Read the model definition and answer for the solid it produces. Units are mm, in the model's axes. A direction names the side the tool comes from. Coordinates: 2 decimals unless noted, no trailing zeros. Loops run counter-clockwise (first coordinate to the right, second up) from the corner with the lowest first, then second, coordinate; pieces in that order, holes last. Notation, with made-up numbers: (-18, 34.5) - (31, 34.5) arc R22 ccw to (31, 65.5) - close; hole circle Ø2 at (-6.75, -15). An arc over 180 degrees is marked (long way). Use one line per item in the form item = value. Start each with the question number.
1) A cutting plane is placed at C-C (z = 2.75). Give the vertices of the cut face in (x, y), and give its area (3 significant figures).
2) The mould has two halves that part along Y. Classify faces 4 (the face through (1, -1, 6.1)), 5 (the face through (-5.158, -3.955, 2.613)), 6 (the face through (0, -1, 3)): released by +Y, released by -Y, zero draft, split by the parting line, or undercut.
3) A cutting plane is placed at A-A (y = 0). Give the vertices of the cut face in (x, z).
4) Consider line 1 (Y direction, x = 0, z = 4); line 2 (Z direction, x = 2, y = -4.5); line 3 (X direction, y = 4.75, z = 1.5). Determine where each line is inside the solid, lowest interval first.
5) A cutting plane is placed at D-D (x = -5). Give the vertices of the cut face in (y, z), and give its area (3 significant figures).
6) Which of the six approach directions +Z, -Z, +X, -X, +Y, -Y give full straight-line access (tool end or side, diameter ignored) to faces 1 (the face through (3, 3, 0)), 2 (the face through (3, 3, 5.3)), 3 (the face through (1, 1, -0.8))?
7) Each of these flat-tipped pins is pushed along its axis until it touches: P1, Ø3, axis at x = 4, y = -3, coming from the +Z side; P2, Ø1, axis at x = 4.5, y = 1, coming from the -Z side; P3, Ø2, axis at x = 4, y = -5, coming from the +Z side. Where does it stop, or does it pass through?
from build123d import *

# Parameters (mm, degrees)
F0_R       = 6.5
F1_DEPTH   = 5.3
F2_R       = 4
F3_DEPTH   = 0.8
F4_R       = 4
F5_DEPTH   = 0.8
F6_SIZE2   = 0.6
F6_SIZE    = 2
F6_2_SIZE2 = 0.6
F6_2_SIZE  = 2
F7_R       = 1
F8_DEPTH   = 6.9


with BuildPart() as f1:
    # F0 (on Top) → F1 (new body)
    with BuildSketch(Plane.XY):
        Circle(F0_R)
    extrude(amount=F1_DEPTH)

    # F2 (on face) → F3 (join)
    with BuildSketch(Plane.XY.offset(5.3)):
        Circle(F2_R)
    extrude(amount=F3_DEPTH)

    # F4 (on face) → F5 (join)
    with BuildSketch(Plane(origin=(0, 0, 0), x_dir=(1, 0, 0), z_dir=(0, 0, -1))):
        Circle(F4_R)
    extrude(amount=F5_DEPTH)

    # F6
    f6_edges = [f1.edges().sort_by_distance(p)[0] for p in [
        (-4, 0, -0.8),
    ]]
    f6_side = f1.faces().sort_by_distance((0, 0, -0.8))[0]
    chamfer(f6_edges, length=F6_SIZE, length2=F6_SIZE2, reference=f6_side)

    # F6#2
    f6_2_edges = [f1.edges().sort_by_distance(p)[0] for p in [
        (-4, 0, 6.1),
    ]]
    f6_2_side = f1.faces().sort_by_distance((0, 0, 6.1))[0]
    chamfer(f6_2_edges, length=F6_2_SIZE, length2=F6_2_SIZE2, reference=f6_2_side)

    # F7 (on face) → F8 (cut, through all)
    with BuildSketch(Plane.XY.offset(6.1)):
        Circle(F7_R)
    extrude(amount=-F8_DEPTH, mode=Mode.SUBTRACT)


solid = f1.part
Found:
q1.outline = circle Ø13 at (0, 0); hole circle Ø2 at (0, 0)
q1.area = 130 mm^2
q2.face_4 = zero draft
q2.face_5 = split by the parting line
q2.face_6 = undercut
q3.outline = (-6.5, 0) - (-4, 0) - (-4, -0.2) - (-2, -0.8) - (-1, -0.8) - (-1, 6.1) - (-2, 6.1) - (-4, 5.5) - (-4, 5.3) - (-6.5, 5.3) - close; (1, -0.8) - (2, -0.8) - (4, -0.2) - (4, 0) - (6.5, 0) - (6.5, 5.3) - (4, 5.3) - (4, 5.5) - (2, 6.1) - (1, 6.1) - close
q4.line_1 = -6.5 to -1, 1 to 6.5
q4.line_2 = 0 to 5.3
q4.line_3 = -4.44 to 4.44
q5.outline = (-4.15, 0) - (4.15, 0) - (4.15, 5.3) - (-4.15, 5.3) - close
q5.area = 44.0 mm^2
q6.face_1 = -Z
q6.face_2 = +Z
q6.face_3 = -Z, +X, -X, +Y, -Y
q7.P1 = 5.65
q7.P2 = 0
q7.P3 = 5.3
